The listing builds one solid part. Answer for the finished solid, in the listing's coordinates (mm). A direction names the side the tool comes from. Coordinates: 2 decimals unless noted, no trailing zeros. Write each loop counter-clockwise with the first axis right and the second up, starting at its lowest first coordinate (ties: lowest second). Pieces come first, ordered by that corner, then holes.
from build123d import *

# Parameters (mm, degrees)
SKETCH_1_R      = 3.4
SKETCH_1_W      = 4.15
SKETCH_1_H      = 4.15
EXTRUDE_1_DEPTH = 600
FILLET_1_R      = 0.7
FILLET_2_R      = 2
FILLET_3_R      = 5


with BuildPart() as part:
    # 草图1 → 凸台-拉伸1 (new body)
    with BuildSketch(Plane(origin=(0, 0, 0), x_dir=(1, 0, 0), z_dir=(0, 1, 0))):
        Polygon((-30, 30), (-19.2, 30), (-19.2, 28), (-23.25, 28), (-23.25, 24.169238816), (-19.080761184, 20), (-10.919238816, 20), (-6.75, 24.169238816), (-6.75, 28), (-10.8, 28), (-10.8, 30), (10.8, 30), (10.8, 28), (6.75, 28), (6.75, 24.169238816), (10.919238816, 20), (19.080761184, 20), (23.25, 24.169238816), (23.25, 28), (19.2, 28), (19.2, 30), (30, 30), (30, 19.2), (28, 19.2), (28, 23.25), (24.169238816, 23.25), (20, 19.080761184), (20, 10.919238816), (24.169238816, 6.75), (28, 6.75), (28, 10.8), (30, 10.8), (30, -10.8), (28, -10.8), (28, -6.75), (24.169238816, -6.75), (20, -10.919238816), (20, -19.080761184), (24.169238816, -23.25), (28, -23.25), (28, -19.2), (30, -19.2), (30, -30), (19.2, -30), (19.2, -28), (23.25, -28), (23.25, -24.169238816), (19.080761184, -20), (10.919238816, -20), (6.75, -24.169238816), (6.75, -28), (10.8, -28), (10.8, -30), (-10.8, -30), (-10.8, -28), (-6.75, -28), (-6.75, -24.169238816), (-10.919238816, -20), (-19.080761184, -20), (-23.25, -24.169238816), (-23.25, -28), (-19.2, -28), (-19.2, -30), (-30, -30), (-30, -19.2), (-28, -19.2), (-28, -23.25), (-24.169238816, -23.25), (-20, -19.080761184), (-20, -10.919238816), (-24.169238816, -6.75), (-28, -6.75), (-28, -10.8), (-30, -10.8), (-30, 10.8), (-28, 10.8), (-28, 6.75), (-24.169238816, 6.75), (-20, 10.919238816), (-20, 19.080761184), (-24.169238816, 23.25), (-28, 23.25), (-28, 19.2), (-30, 19.2), align=None)
        with Locations(Location((-15, 15, 0), (0, 0, 270))):
            Circle(SKETCH_1_R, mode=Mode.SUBTRACT)
        with Locations(Location((15, 15, 0), (0, 0, 270))):
            Circle(SKETCH_1_R, mode=Mode.SUBTRACT)
        with Locations(Location((15, -15, 0), (0, 0, 270))):
            Circle(SKETCH_1_R, mode=Mode.SUBTRACT)
        with Locations(Location((-15, -15, 0), (0, 0, 270))):
            Circle(SKETCH_1_R, mode=Mode.SUBTRACT)
        Polygon((-5.45, 28), (-5.45, 28.7), (5.45, 28.7), (5.45, 28), (5.45, 23.630761184), (10, 19.080761184), (10, 10), (19.080761184, 10), (23.630761184, 5.45), (28, 5.45), (28.7, 5.45), (28.7, -5.45), (28, -5.45), (23.630761184, -5.45), (19.080761184, -10), (10, -10), (10, -19.080761184), (5.45, -23.630761184), (5.45, -28), (5.45, -28.7), (-5.45, -28.7), (-5.45, -28), (-5.45, -23.630761184), (-10, -19.080761184), (-10, -10), (-19.080761184, -10), (-23.630761184, -5.45), (-28, -5.45), (-28.7, -5.45), (-28.7, 5.45), (-28, 5.45), (-23.630761184, 5.45), (-19.080761184, 10), (-10, 10), (-10, 19.080761184), (-5.45, 23.630761184), align=None, mode=Mode.SUBTRACT)
        with Locations((-26.625, 26.625)):
            Rectangle(SKETCH_1_W, SKETCH_1_H, mode=Mode.SUBTRACT)
        with Locations((26.625, 26.625)):
            Rectangle(SKETCH_1_W, SKETCH_1_H, mode=Mode.SUBTRACT)
        with Locations((26.625, -26.625)):
            Rectangle(SKETCH_1_W, SKETCH_1_H, mode=Mode.SUBTRACT)
        with Locations((-26.625, -26.625)):
            Rectangle(SKETCH_1_W, SKETCH_1_H, mode=Mode.SUBTRACT)
    extrude(amount=EXTRUDE_1_DEPTH)

    # 圆角1
    fillet_1_edges = [part.edges().sort_by_distance(p)[0] for p in [
        (28.7, 300, 28.7),
        (28.7, 300, -28.7),
        (-28.7, 300, -28.7),
        (-28.7, 300, 28.7),
    ]]
    fillet(fillet_1_edges, radius=FILLET_1_R)

    # 圆角2
    fillet_2_edges = [part.edges().sort_by_distance(p)[0] for p in [
        (30, 300, -30),
        (30, 300, 30),
        (-30, 300, 30),
        (-30, 300, -30),
    ]]
    fillet(fillet_2_edges, radius=FILLET_2_R)

    # 圆角3
    fillet_3_edges = [part.edges().sort_by_distance(p)[0] for p in [
        (10, 300, 10),
        (10, 300, -10),
        (-10, 300, -10),
        (-10, 300, 10),
    ]]
    fillet(fillet_3_edges, radius=FILLET_3_R)


solid = part.part
Q1. Determine the mould class of faces 1 (the face through (-30, 296, 0)), 2 (the face through (0, 296, 30)), 3 (the face through (28.7, 296, 0)), 4 (the face through (-28.7, 296, 0)) for opening direction X: released by +X, released by -X, zero draft, split by the parting line, or undercut.
Answers below:
face 1: released by -X
face 2: zero draft
face 3: undercut
face 4: undercut
Q2. The part is cut by section B-B, the plane y = 143.5. State how many separate pieces and enclosed holes the cut face has, then the cut area to 3 significant figures.
Answers below:
separate pieces: 1
enclosed holes: 9
area: 681 mm2
Q3. The part is cut by section A-A, the plane x = 0.5. Write down the section's boundary in (y, z), then the cut area to 3 significant figures.
Answers below:
outline: (0, -30) - (600, -30) - (600, -28.7) - (0, -28.7) - close; (0, 28.7) - (600, 28.7) - (600, 30) - (0, 30) - close
area: 1,560 mm2
Q4. Find the intervals of material crossed by probe 1 along X at (y, z) = (392, 15); probe 2 along Z at (x, y) = (4, 103.5); probe 3 along Z at (x, y) = (-5.5, 555), in increasing order.
Answers below:
probe 1: x = -20 to -18.4, -11.6 to -10, 10 to 11.6, 18.4 to 20
probe 2: z = -30 to -28.7, 28.7 to 30
probe 3: z = -30 to -23.58, 23.58 to 30
Q5. Given pin 1 (2 mm diameter, centred on x = 29.5, y = 364.5, fed in from +Z); pin 2 (1.6 mm diameter, centred on y = 437.5, z = 29, fed in from -X); pin 3 (1.5 mm diameter, centred on x = -16.5, y = 278, fed in from -Z), each flat-ended and moving along its own axis, determine where each tip first touches the part or whether it passes through.
Answers below:
pin 1: stops at z = 29.94
pin 2: stops at x = -29.99
pin 3: stops at z = -20
Q6. Which of the six approach directions +Z, -Z, +X, -X, +Y, -Y give full straight-line access (tool end or side, diameter ignored) to faces 5 (the face through (0, 296, 28.7)), 6 (the face through (30, 296, 0))?
Answers below:
face 5: +Y, -Y
face 6: +Z, -Z, +X, +Y, -Y
